from build123d import *

# Parameters (mm, degrees)
SKETCH002_R     = 19
SKETCH003_R     = 20
PAD_DEPTH       = 2
SKETCH005_R     = 19
POCKET_DEPTH    = 2
SKETCH006_R     = 1.5
POCKET001_DEPTH = 5


with BuildPart() as loft_body:
    # Sketch → Loft section 0
    with BuildSketch(Plane.XY):
        with BuildLine():
            ThreePointArc((-16, 3), (-19, 0), (-16, -3))
            Line((-16, -3), (16, -3))
            ThreePointArc((16, -3), (19, 0), (16, 3))
            Line((-16, 3), (16, 3))
        make_face()
    # Sketch002 → Loft section 1
    with BuildSketch(Plane.XY.offset(17)):
        Circle(SKETCH002_R)
    loft()


with BuildPart() as pocket001:
    # Sketch001 → Loft001 section 0
    with BuildSketch(Plane.XY):
        with BuildLine():
            ThreePointArc((-16, 4), (-20, 0), (-16, -4))
            Line((-16, -4), (16, -4))
            ThreePointArc((16, -4), (20, 0), (16, 4))
            Line((-16, 4), (16, 4))
        make_face()
    # Sketch003 → Loft001 section 1
    with BuildSketch(Plane.XY.offset(17)):
        Circle(SKETCH003_R)
    loft()

    # Cut: cut Loft body
    add(loft_body.part, mode=Mode.SUBTRACT)

    # Sketch004 → Pad (new body)
    with BuildSketch(Plane.XY.offset(17)):
        with BuildLine():
            Line((-18, 20), (18, 20))
            ThreePointArc((20, 18), (19.414214, 19.414214), (18, 20))
            Line((20, 18), (20, -18))
            ThreePointArc((18, -20), (19.414214, -19.414214), (20, -18))
            Line((18, -20), (-18, -20))
            ThreePointArc((-20, -18), (-19.414214, -19.414214), (-18, -20))
            Line((-20, -18), (-20, 18))
            ThreePointArc((-18, 20), (-19.414214, 19.414214), (-20, 18))
        make_face()
    extrude(amount=PAD_DEPTH)

    # Sketch005 → Pocket (cut)
    with BuildSketch(Plane.XY.offset(19)):
        Circle(SKETCH005_R)
    extrude(amount=-POCKET_DEPTH, mode=Mode.SUBTRACT)

    # Sketch006 → Pocket001 (cut)
    with BuildSketch(Plane.XY.offset(19)):
        with Locations((-16, 16)):
            Circle(SKETCH006_R)
        with Locations((16, 16)):
            Circle(SKETCH006_R)
        with Locations((-16, -16)):
            Circle(SKETCH006_R)
        with Locations((16, -16)):
            Circle(SKETCH006_R)
    extrude(amount=-POCKET001_DEPTH, mode=Mode.SUBTRACT)


solid = pocket001.part
For this review, take the finished solid that the model builds, in its own axes (mm). A direction names the side the tool comes from. Round coordinates to 2 decimals unless told otherwise and drop trailing zeros. Write item = value, one per line. Start each with the question number.
1. For faces 1 (the face through (15, 14, 17)), 2 (the face through (-14, 16, 17)), 3 (the face through (-14, -16, 17)), list the 3-axis set-ups (+Z, -Z, +X, -X, +Y, -Y) from which the entire face can be reached by the end or side of a thin tool; tool diameter is ignored.
2. Consider section A-A on y = 17. Give the number of separate pieces and of enclosed holes in the cut face, plus the area to 3 significant figures.
3. For pin 1 Ø1.5 at (x, z) = (0, 14) entering from +Y; pin 2 Ø5 at (x, z) = (4, 13.5) entering from +Y; pin 3 Ø1.5 at (x, z) = (11, 4) entering from +Y, all flat-tipped, find the tip position at first contact; note any pin that passes through.
4. Wall thickness on L1, parallel to X at y = 0, z = 18.2; L2, parallel to Y at x = 16, z = 18.3; L3, parallel to Y at x = 5, z = 12: over which ranges is each line inside the solid? List them lowest first.
5. Draft analysis for pull direction Y (two halves, no side actions). For faces 4 (the face through (0, -20, 18)), 5 (the face through (8.767, -16.856, 18.014)), 6 (the face through (14.5, -15.93, 18.01)), 7 (the face through (20, 0, 18)), state which applies: released by +Y, released by -Y, zero draft, split by the parting line, or undercut.
Evaluation:
q1.face_1 = -Z, +X, +Y
q1.face_2 = -Z, -X, +Y
q1.face_3 = -Z, -X, -Y
q2.separate_pieces = 3
q2.enclosed_holes = 0
q2.area = 58.6 mm2
q3.pin_1 = 17.88
q3.pin_2 = 18.71
q3.pin_3 = 6.82
q4.L1 = -20 to -19, 19 to 20
q4.L2 = -20 to -17.5, -14.5 to -10.25, 10.25 to 14.5, 17.5 to 20
q4.L3 = -14.72 to -13.69, 13.69 to 14.72
q5.face_4 = released by -Y
q5.face_5 = undercut
q5.face_6 = undercut
q5.face_7 = zero draft
